Autodesk Inventor part; units mm, degrees
ref_plane "YZ Plane" through (0, 0, 0) normal (1, 0, 0) x (0, 1, 0)
ref_plane "XZ Plane" through (0, 0, 0) normal (0, 1, 0) x (-1, 0, 0)
ref_plane "XY Plane" through (0, 0, 0) normal (0, 0, 1) x (1, 0, 0)
sketch "Sketch1" plane through (0, 0, 0) normal (0, 0, 1) x (1, 0, 0)
  circle A0 centre (7.8339, 40) radius 4.5
  circle A1 centre (7.8339, 40) radius 1.5
  circle A2 centre (9.4447, 20) radius 4.5
  circle A3 centre (9.4447, 20) radius 1.5
  circle A4 centre (34.6118, -20) radius 4.5
  circle A5 centre (34.6118, -20) radius 1.5
  circle A6 centre (53.9309, -32) radius 4.5
  circle A7 centre (53.9309, -32) radius 1.5
  line L0 (3.3484, 39.6387) -> (4.9593, 19.6387)
  circle A8 centre (35, 0) radius 7.025
  line L1 (6.404, 16.6828) -> (26.106, -1.3771)
  line L2 (28.617, -6.3449) -> (30.1377, -20.4813)
  line L3 (32.2374, -23.8226) -> (51.5565, -35.8226)
  circle A9 centre (35, 0) radius 4.025
  line L4 (14.3908, 21.5707) -> (31.3649, 6.0114)
  arc A10 (14.3908, 21.5707) -> (11.951, 41.8166) centre (-20.0705, 27.6877) ccw
  arc A11 (57.4046, -29.1394) -> (41.0725, -17.3055) centre (26.5269, -54.5671) ccw
  arc A12 (41.0725, -17.3055) -> (42.0194, 0.2811) centre (-51.9053, -3.4806) ccw
  arc A13 (26.106, -1.3771) -> (28.617, -6.3449) centre (35, 0) ccw
  dimension "d9" = 14.05
  dimension "d10" = 8.05
  dimension "d11" = 35
  dimension "d12" = 40
  dimension "d13" = 94
  dimension "d15" = 7
extrude "Extrusion1" add sketch "Sketch1" against normal blind 3
fillet "Fillet1" radius 2 5 edges at (26.106, -1.3771, -1.5) (28.617, -6.3449, -1.5) (14.3908, 21.5707, -1.5) (41.0725, -17.3055, -1.5) (31.3649, 6.0114, -1.5)
properties part number "アーノン" material "Aluminum 7075"
Can you work these out from the model? Positions are in its coordinate system, mm. Give positions to 0.01 mm unless a question says otherwise; leave off trailing zeros. Order: outer loops, then holes, each group sorted by start corner. A loop starts at its lowest first (then second) coordinate and runs counter-clockwise, first axis right, second up. Notation, with made-up numbers: M 76,-5.75 L 95,-5.75 A23 ccw 95,2.25 Z; hole C 25.5,61 d8. An arc over 180 degrees is marked long. One line per item, written item: value.
Item 1: If we section it at C-C on y = -32: Write out the boundary of the cut face in (x, z), and give its area (3 significant figures).
Verdict:
outline: M 45.4,-3 L 52.43,-3 L 52.43,0 L 45.4,0 Z; M 55.43,-3 L 58.43,-3 L 58.43,0 L 55.43,0 Z
area: 30.1 mm2
Item 2: Please list where these lines run through material, in increasing order: line 1 (X direction, y = -19, z = -0.8); line 2 (Y direction, x = 36.5, z = -2); line 3 (X direction, y = -9, z = -0.6).
Verdict:
line 1: 29.98 to 33.49, 35.73 to 44.83
line 2: -26.47 to -3.74, 3.74 to 6.86
line 3: 28.9 to 41.93
Item 3: If we section it at D-D on z = -2.5: State how many separate pieces and enclosed holes the cut face has, and give its area (3 significant figures).
Verdict:
separate pieces: 1
enclosed holes: 5
area: 990 mm2
Item 4: For pin 1 (1.8 mm diameter, centred on x = 34.61, y = -20, fed in from +Z), with a flat end and sliding along its axis, tell me the tip position at first contact or that it passes through.
Verdict:
pin 1: through
Item 5: If we section it at A-A on y = -3: Write out the boundary of the cut face in (x, z), and give its area (3 significant figures).
Verdict:
outline: M 26.51,-3 L 32.32,-3 L 32.32,0 L 26.51,0 Z; M 37.68,-3 L 42.09,-3 L 42.09,0 L 37.68,0 Z
area: 30.6 mm2
Item 6: If we mould it in two halves opening along Y, with no side actions, what happens to faces 1 (the face through (26.954, -4.032, -1.479)), 2 (the face through (38.92, 5.83, -1.48)), 3 (the face through (41.99, -7.88, -1.48))? For each: pulls with the +Y half, pulls with the -Y half, needs draft (parallel to the pull), parting line crosses it, or undercut.
Verdict:
face 1: pulls with the -Y half
face 2: pulls with the +Y half
face 3: undercut
Item 7: If we section it at B-B on x = 35: Write out the boundary of the cut face in (y, z) (3 decimals).
Verdict:
outline: M -25.539,-3 L -21.449,-3 L -21.449,0 L -25.539,0 Z; M -18.551,-3 L -4.025,-3 L -4.025,0 L -18.551,0 Z; M 4.025,-3 L 7.025,-3 L 7.025,0 L 4.025,0 Z
